```python
from build123d import *

# Parameters (mm, degrees)
SKETCH1_R           = 1.125
SKETCH1_R_2         = 0.15
BOSS_EXTRUDE1_DEPTH = 7
SKETCH2_R           = 4
SKETCH2_R_2         = 1.125
BOSS_EXTRUDE2_DEPTH = 0.2
CHAMFER1_SIZE       = 0.2


with BuildPart() as part:
    # Sketch1 → Boss-Extrude1 (new body)
    with BuildSketch(Plane.XY):
        Circle(SKETCH1_R)
        Circle(SKETCH1_R_2, mode=Mode.SUBTRACT)
    extrude(amount=BOSS_EXTRUDE1_DEPTH)

    # Sketch2 → Boss-Extrude2 (add)
    with BuildSketch(Plane.XY.offset(7)):
        with Locations((0.018669882, 0)):
            Circle(SKETCH2_R)
        Circle(SKETCH2_R_2, mode=Mode.SUBTRACT)
    extrude(amount=-BOSS_EXTRUDE2_DEPTH)

    # Chamfer1
    chamfer1_edges = [part.edges().sort_by_distance(p)[0] for p in [
        (-1.125, 0, 0),
        (-0.15, 0, 0),
        (-0.15, 0, 7),
    ]]
    chamfer(chamfer1_edges, length=CHAMFER1_SIZE)


solid = part.part
```
For this review, take the finished solid that the model builds, in its own axes (mm). A direction names the side the tool comes from. Round coordinates to 2 decimals unless told otherwise and drop trailing zeros. Order: outer loops, then holes, each group sorted by start corner. A loop starts at its lowest first (then second) coordinate and runs counter-clockwise, first axis right, second up. Notation, with made-up numbers: (29.5, 79) -> (37.5, 79) arc R17 ccw to (37.5, 83) -> close; hole circle Ø1 at (62, -9). An arc over 180 degrees is marked (long way). Use a Markdown table: item, result.
Item 1: Machinability: for faces 1 (the flat face through (0, -1, 7)), 2 (the cylindrical face through (-0.146, 1.115, 3.454)), which of the approach directions +Z, -Z, +X, -X, +Y, -Y give a long, thin tool a straight path to every point of the face, cutting with its end or side? Answer none if there is none.
Resolved:
| item | result |
|---|---|
| face 1 | +Z, +X, -X, +Y, -Y |
| face 2 | -Z |
Item 2: Take a section at A-A (y = 0). State the section outline as (x, z) points (3 decimals).
Resolved:
| item | result |
|---|---|
| outline | (-3.981, 6.8) -> (-1.125, 6.8) -> (-1.125, 0.2) -> (-0.925, 0) -> (-0.35, 0) -> (-0.15, 0.2) -> (-0.15, 6.8) -> (-0.35, 7) -> (-3.981, 7) -> close; (0.15, 0.2) -> (0.35, 0) -> (0.925, 0) -> (1.125, 0.2) -> (1.125, 6.8) -> (4.019, 6.8) -> (4.019, 7) -> (0.35, 7) -> (0.15, 6.8) -> close |
Item 3: For line 1 along Y through (x, z) = (0, 2.5) (3 decimals); line 2 along Z through (x, y) = (0.5, 2.5); line 3 along Y through (x, z) = (1, 2.5), list the stretches that pass through material, from the lowest coordinate up. Write a range as [from, to].
Resolved:
| item | result |
|---|---|
| line 1 | y = [-1.125, -0.15], [0.15, 1.125] |
| line 2 | z = [6.8, 7] |
| line 3 | y = [-0.52, 0.52] |
Item 4: Take a section at D-D (x = -3). State the section outline as (y, z) points.
Resolved:
| item | result |
|---|---|
| outline | (-2.62, 6.8) -> (2.62, 6.8) -> (2.62, 7) -> (-2.62, 7) -> close |
Item 5: For pin 1 (4 mm diameter, centred on x = 2.5, z = 4, fed in from +Y); pin 2 (3 mm diameter, centred on x = -3, y = -1.5, fed in from -Z); pin 3 (2 mm diameter, centred on y = 1, z = 1, fed in from +X) (3 decimals), all flat-tipped, find the tip position at first contact; note any pin that passes through.
Resolved:
| item | result |
|---|---|
| pin 1 | stops at y = 1.01 |
| pin 2 | stops at z = 6.8 |
| pin 3 | stops at x = 1.125 |
Item 6: Take a section at C-C (z = 3.5). State the section outline as (x, y) points (3 decimals).
Resolved:
| item | result |
|---|---|
| outline | circle Ø2.25 at (0, 0); hole circle Ø0.3 at (0, 0) |
Item 7: Take a section at B-B (x = 0). State the section outline as (y, z) points (3 decimals), plus the area to 3 significant figures.
Resolved:
| item | result |
|---|---|
| outline | (-4, 6.8) -> (-1.125, 6.8) -> (-1.125, 0.2) -> (-0.925, 0) -> (-0.35, 0) -> (-0.15, 0.2) -> (-0.15, 6.8) -> (-0.35, 7) -> (-4, 7) -> close; (0.15, 0.2) -> (0.35, 0) -> (0.925, 0) -> (1.125, 0.2) -> (1.125, 6.8) -> (4, 6.8) -> (4, 7) -> (0.35, 7) -> (0.15, 6.8) -> close |
| area | 14.7 mm² |
